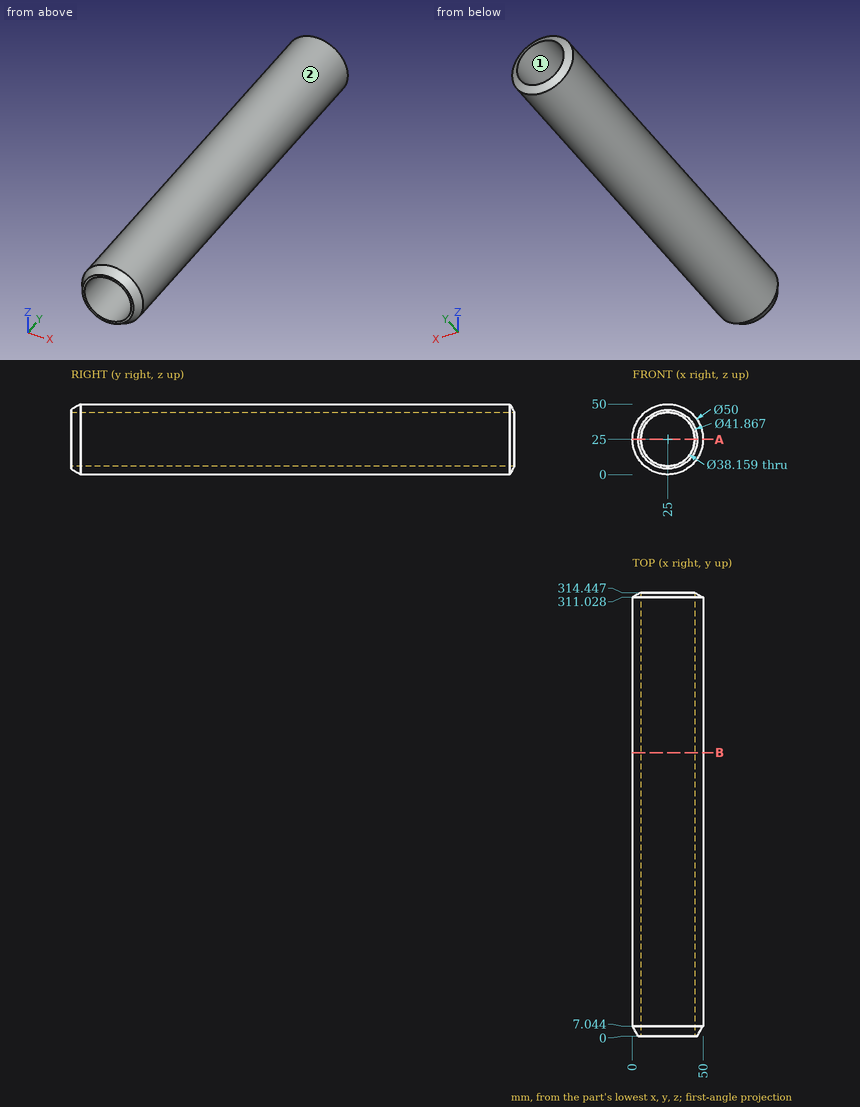
Study the drawing (mm; zero at the part's minimum x, y, z) and answer. Give positions to 0.01 mm unless a question says otherwise; leave off trailing zeros. Loops run counter-clockwise (first coordinate to the right, second up) from the corner with the lowest first, then second, coordinate; pieces in that order, holes last. Notation, with made-up numbers: (-33, -16.5) - (-17, -16.5) arc R19 ccw to (-17, -7.5) - close; hole circle Ø9 at (8.25, 55.25). An arc over 180 degrees is marked (long way). One line per question, with ' | ' between items.
(1) The part is cut by section B-B (y = 201). Write down the section's boundary in (x, z), then the cut area to 3 significant figures.
Recorded:
outline: circle Ø50 at (25, 25); hole circle Ø38.16 at (25, 25) | area: 820 mm²
(2) Each of these flat-tipped pins is pushed along its axis until it touches: pin 1 Ø2 at (y, z) = (274, 26.5) entering from +X (1 decimal); pin 2 Ø5 at (x, y) = (27, 70.5) entering from +Z; pin 3 Ø12 at (y, z) = (205.5, 30) entering from -X; pin 4 Ø1 at (y, z) = (58, 8.5) entering from +X. Where does it stop, or does it pass through?
Recorded:
pin 1: stops at x = 50 | pin 2: stops at z = 50 | pin 3: stops at x = 0 | pin 4: stops at x = 44.21
(3) Straight lines are drawn through the part: probe 1 along X at (y, z) = (69.5, 25); probe 2 along X at (y, z) = (30, 38) (1 decimal); probe 3 along Z at (x, y) = (41, 28) (1 decimal). For each, find the intervals that lie inside material, in ascending order.
Recorded:
probe 1: x = 0 to 5.92, 44.08 to 50 | probe 2: x = 3.6 to 11, 39 to 46.4 | probe 3: z = 5.8 to 14.6, 35.4 to 44.2
(4) The part is cut by section A-A (z = 25). Write down the section's boundary in (x, y).
Recorded:
outline: (0, 7.04) - (4.07, 0) - (5.92, 0) - (5.92, 314.45) - (0, 311.03) - close; (44.08, 0) - (45.93, 0) - (50, 7.04) - (50, 311.03) - (44.08, 314.45) - close
(5) The mould has two halves that part along Z. Classify the marked faces 1 and 2: +Z half, -Z half, draft (parallel to the pull), parting line (faces both ways), or undercut.
Recorded:
face 1: undercut | face 2: parting line
